Source: CAD feature listing. Evaluate the final solid. Frame: model axes, mm. A direction names the side the tool comes from. Round coordinates to 2 decimals unless told otherwise and drop trailing zeros. Order: outer loops, then holes, each group sorted by start corner. A loop starts at its lowest first (then second) coordinate and runs counter-clockwise, first axis right, second up. Notation, with made-up numbers: M 86.5,77 L 127.5,77 A7 cw 127.5,83 Z; hole C -18,31 d10. An arc over 180 degrees is marked long. Use one line per item in the form item = value. Start each with the question number.
Q1. Pull-direction query (Z, two-part tool) for faces 1 (the flat face through (5, -8, -26)), 2 (the cylindrical face through (29.082, 6.92, -10.783)), 3 (the flat face through (11, -7, 25)), 4 (the cylindrical face through (11.31, -7.6, -30.63)); classes: pulls with the +Z half, pulls with the -Z half, needs draft (parallel to the pull), parting line crosses it, or undercut.
Q2. Section B-B (z = 18). Return the cut outline in (x, y), plus the area to 3 significant figures.
Q3. Reachability of faces 5 (the cylindrical face through (29.082, 7.215, 10.58)), 6 (the flat face through (17, -6.309, -20)), 7 (the cylindrical face through (8.926, 5.022, 20.766)), 8 (the flat face through (11, -9, 19.08)), 9 (the conical face through (-6.188, 6.383, 1.487)) from +Z, -Z, +X, -X, +Y, -Y: full face, straight path, thin tool, end or side. Return the list, or none.
Q4. Section A-A (x = 19). Give the number of separate pieces and of enclosed holes in the cut face, plus the area to 3 significant figures.
Q5. Contact query for flat-ended pins moving along their axis: pin 1 (8 mm diameter, centred on x = 20.5, z = 3, fed in from -Y); pin 2 (4 mm diameter, centred on x = 16.5, z = 25.5, fed in from +Y); pin 3 (7 mm diameter, centred on y = -1.5, z = 3.5, fed in from -X); pin 4 (3 mm diameter, centred on y = 0.5, z = 15.5, fed in from +X). Output: stop coordinate, or through.
Q6. Material intervals for probe 1 along X at (y, z) = (1, 6.5); probe 2 along X at (y, z) = (7.5, -6); probe 3 along Z at (x, y) = (14, 7), sorted ascending.
from build123d import *

# Parameters (mm, degrees)
BOSS_EXTRUDE1_DEPTH     = 22.3
SKETCH4_R               = 2.5
CUT_EXTRUDE1_DEPTH      = 1
SKETCH5_R               = 0.5
CUT_EXTRUDE2_DEPTH      = 49.261993328
CUT_EXTRUDE3_DEPTH      = 14.8
FILLET1_R               = 5
BOSS_EXTRUDE2_DEPTH     = 9
FILLET2_R               = 2
FILLET3_R               = 5
SKETCH11_R              = 3.065
BOSS_EXTRUDE3_DEPTH     = 4.5
SKETCH12_R              = 8.5
CUT_EXTRUDE4_DEPTH      = 3
CUT_EXTRUDE4_DRAFT      = -30
MIRROR5_COPY_1_SKETCH_R = 8.5
MIRROR5_COPY_1_DEPTH    = 3
MIRROR5_COPY_1_DRAFT    = -30


# Read off the part's stored shape, not the designer's step: Boss-Extrude2
with BuildPart() as part:
    # Sketch2 → Boss-Extrude1 (new body)
    with BuildSketch(Plane(origin=(0, 0, 0), x_dir=(0, 0, -1), z_dir=(1, 0, 0))):
        with BuildLine():
            Line((-19.08, -7), (-19.08, -10))
            Line((-19.08, -10), (-31.2, -10))
            Line((-31.2, -10), (-31.2, -7))
            Line((-31.2, -7), (-21.2, -7))
            ThreePointArc((-21.2, -7), (-18.082442737, 13.063917612), (0, 22.3))
            ThreePointArc((0, 22.3), (18.082442737, 13.063917612), (21.2, -7))
            Line((21.2, -7), (31.2, -7))
            Line((31.2, -7), (31.2, -10))
            Line((31.2, -10), (19.08, -10))
            Line((19.08, -10), (19.08, -7))
            ThreePointArc((19.08, -7), (16.651833626, 11.620468336), (0, 20.3))
            ThreePointArc((0, 20.3), (-16.651833626, 11.620468336), (-19.08, -7))
        make_face()
    extrude(amount=BOSS_EXTRUDE1_DEPTH)

    # Sketch4 → Cut-Extrude1 (cut)
    with BuildSketch(Plane(origin=(0, -7, 0), x_dir=(1, 0, 0), z_dir=(0, 1, 0))):
        with Locations(Location((5, 26.695, 0), (0, 0, 270))):
            Circle(SKETCH4_R)
        with Locations(Location((17.3, 26.695, 0), (0, 0, 270))):
            Circle(SKETCH4_R)
        with Locations(Location((5, -26.695, 0), (0, 0, 270))):
            Circle(SKETCH4_R)
        with Locations(Location((17.3, -26.695, 0), (0, 0, 270))):
            Circle(SKETCH4_R)
    extrude(amount=-CUT_EXTRUDE1_DEPTH, mode=Mode.SUBTRACT)

    # Sketch5 → Cut-Extrude2 (cut, through all)
    with BuildSketch(Plane(origin=(0, -7, 0), x_dir=(1, 0, 0), z_dir=(0, 1, 0))):
        with Locations(Location((17.3, 26.695, 0), (0, 0, 270))):
            Circle(SKETCH5_R)
        with Locations(Location((5, 26.695, 0), (0, 0, 270))):
            Circle(SKETCH5_R)
        with Locations(Location((5, -26.695, 0), (0, 0, 270))):
            Circle(SKETCH5_R)
        with Locations(Location((17.3, -26.695, 0), (0, 0, 270))):
            Circle(SKETCH5_R)
    extrude(amount=-CUT_EXTRUDE2_DEPTH, mode=Mode.SUBTRACT)

    # Sketch6 → Cut-Extrude3 (cut)
    with BuildSketch(Plane(origin=(22.3, 0, 0), x_dir=(0, 0, -1), z_dir=(1, 0, 0))):
        Polygon((0, 0), (46.533038178, 14.787970064), (46.533038178, -6.309411423), (19, -6.309411423), align=None)
    cut_extrude3 = extrude(amount=-CUT_EXTRUDE3_DEPTH, mode=Mode.SUBTRACT)

    # Fillet1
    fillet1_edges = [part.edges().sort_by_distance(p)[0] for p in [
        (7.5, 6.454741119, -20.311017239),
        (7.5, -6.309411423, -20.366815992),
    ]]
    fillet(fillet1_edges, radius=FILLET1_R)

    # Boss-Extrude2 outline → Boss-Extrude2 (add)
    with BuildSketch(Plane(origin=(22.3, 0, 0), x_dir=(0, 0, -1), z_dir=(1, 0, 0))):
        with BuildLine():
            Line((-19.08, -10), (-19.08, -7))
            ThreePointArc((-19.08, -7), (-16.651833626, 11.620468336), (0, 20.3))
            ThreePointArc((0, 20.3), (0.00031837, 20.299999942), (0.000636741, 20.299999879))
            ThreePointArc((0.000636741, 20.299999879), (16.65523283, 11.62577033), (19.089327288, -6.993924006))
            Line((19.089327288, -6.993924006), (19.0902824, -9.993923854))
            Line((19.0902824, -9.993923854), (31.210281785, -9.990065204))
            Line((31.210281785, -9.990065204), (31.209326674, -6.990065356))
            Line((31.209326674, -6.990065356), (21.209327181, -6.993249061))
            ThreePointArc((21.209327181, -6.993249061), (18.085382316, 13.069674996), (0, 22.3))
            ThreePointArc((0, 22.3), (-18.082442737, 13.063917612), (-21.2, -7))
            Line((-21.2, -7), (-31.2, -7))
            Line((-31.2, -7), (-31.2, -10))
            Line((-31.2, -10), (-19.08, -10))
        make_face()
    boss_extrude2 = extrude(amount=BOSS_EXTRUDE2_DEPTH)

    # Mirror1: Boss-Extrude2 across plane
    add(boss_extrude2.mirror(Plane(origin=(11.15, 0, 0), x_dir=(0, 0, 1), z_dir=(1, 0, 0))))

    # Fillet2
    fillet2_edges = [part.edges().sort_by_distance(p)[0] for p in [
        (26.8, -6.990065356, -31.209326674),
        (-4.5, -6.990065356, -31.209326674),
        (11.15, -7, 31.2),
        (11.15, -7, -31.2),
    ]]
    fillet(fillet2_edges, radius=FILLET2_R)

    # Mirror2: Cut-Extrude3 across plane
    add(cut_extrude3.mirror(Plane.XY), mode=Mode.SUBTRACT)

    # Fillet3
    fillet3_edges = [part.edges().sort_by_distance(p)[0] for p in [
        (7.5, -6.309411423, 20.366815992),
        (7.5, 6.454741119, 20.311017239),
    ]]
    fillet(fillet3_edges, radius=FILLET3_R)

    # Sketch11 → Boss-Extrude3 (add)
    with BuildSketch(Plane(origin=(31.3, 0, 0), x_dir=(0, 0, -1), z_dir=(1, 0, 0))):
        with BuildLine():
            Line((-19.08, -10), (19.087106029, -10))
            Line((19.087106029, -10), (19.087106029, -7))
            ThreePointArc((19.087106029, -7), (14.745407201, -8.568352102), (11.816765825, -5))
            ThreePointArc((11.816765825, -5), (10.685839373, 7.068100067), (0.005794631, 12.800000115))
            Line((0.005794631, 12.800000115), (0.001311398, 12.800000115))
            ThreePointArc((0.001311398, 12.800000115), (-10.678733344, 7.068100067), (-11.809659796, -5))
            ThreePointArc((-11.809659796, -5), (-14.738301172, -8.568352102), (-19.08, -7))
            Line((-19.08, -7), (-19.08, -10))
        make_face()
        with Locations((0.003553015, -0.329999689)):
            Circle(SKETCH11_R, mode=Mode.SUBTRACT)
    boss_extrude3 = extrude(amount=-BOSS_EXTRUDE3_DEPTH)


with BuildPart() as cut_extrude4_tool:
    # Sketch12 → Cut-Extrude4 (with draft: the straight prism first)
    with BuildSketch(Plane(origin=(31.3, 0, 0), x_dir=(0, 0, -1), z_dir=(1, 0, 0))):
        with Locations((0.003553015, -0.329999689)):
            Circle(SKETCH12_R)
    extrude(amount=-CUT_EXTRUDE4_DEPTH)
    # Cut-Extrude4: the draft: its side faces are tilted about the plane it starts from
    cut_extrude4_sides = [cut_extrude4_tool.faces().sort_by_distance(p)[0] for p in [
        (29.8, -0.329999689, 8.496446985),
    ]]
    draft(cut_extrude4_sides, Plane(origin=(31.3, 0, 0), x_dir=(0, 0, -1), z_dir=(1, 0, 0)), CUT_EXTRUDE4_DRAFT)


with BuildPart() as part_1:
    add(part.part)

    # Cut-Extrude4: cut by cut_extrude4_tool
    add(cut_extrude4_tool.part, mode=Mode.SUBTRACT)

    # Mirror4: Boss-Extrude3 across plane
    add(boss_extrude3.mirror(Plane(origin=(11.15, 0, 0), x_dir=(0, 0, 1), z_dir=(1, 0, 0))))


with BuildPart() as mirror5_copy_1_tool:
    # Mirror5 copy 1 sketch → Mirror5 copy 1 (with draft: the straight prism first)
    with BuildSketch(Plane(origin=(-9, 0, 0), x_dir=(0, 0, -1), z_dir=(-1, 0, 0))):
        with Locations((0.003553015, 0.329999689)):
            Circle(MIRROR5_COPY_1_SKETCH_R)
    extrude(amount=-MIRROR5_COPY_1_DEPTH)
    # Mirror5 copy 1: the draft: its side faces are tilted about the plane it starts from
    mirror5_copy_1_sides = [mirror5_copy_1_tool.faces().sort_by_distance(p)[0] for p in [
        (-7.5, -0.329999689, 8.496446985),
    ]]
    draft(mirror5_copy_1_sides, Plane(origin=(-9, 0, 0), x_dir=(0, 0, -1), z_dir=(-1, 0, 0)), MIRROR5_COPY_1_DRAFT)


with BuildPart() as part_2:
    add(part_1.part)

    # Mirror5 copy 1: cut by mirror5_copy_1_tool
    add(mirror5_copy_1_tool.part, mode=Mode.SUBTRACT)


solid = part_2.part
Results list:
q1.face_1 = undercut
q1.face_2 = undercut
q1.face_3 = needs draft
q1.face_4 = pulls with the -Z half
q2.outline = M -9,-10 L -4.5,-10 L -4.5,-8.05 L -9,-8.05 Z; M -9,9.4 L 31.3,9.4 L 31.3,13.18 L -9,13.18 Z; M 26.8,-10 L 31.3,-10 L 31.3,-8.05 L 26.8,-8.05 Z
q2.area = 170 mm2
q3.face_5 = +X, -X
q3.face_6 = +Z, -Z
q3.face_7 = +Z
q3.face_8 = -Y
q3.face_9 = -X
q4.separate_pieces = 3
q4.enclosed_holes = 0
q4.area = 174 mm2
q5.pin_1 = 19.05
q5.pin_2 = -7
q5.pin_3 = -6.74
q5.pin_4 = through
q6.probe_1 = -6 to -4.5, 26.8 to 28.3
q6.probe_2 = -9 to -4.5, 26.8 to 31.3
q6.probe_3 = -21.19 to -19.07, 19.07 to 21.19
